```python
from build123d import *

# Parameters (mm, degrees)
SKETCH1_W                = 50
SKETCH1_H                = 35.6
BOSS_EXTRUDE2_DEPTH      = 15
SKETCH9_W                = 2.17
SKETCH9_H                = 25.6
CUT_EXTRUDE1_DEPTH       = 10.3
SKETCH7_R                = 1.32
CUT_EXTRUDE2_DEPTH       = 34.770899441
SKETCH10_R               = 0.81
CUT_EXTRUDE3_DEPTH       = 8
BOSS_EXTRUDE3_DEPTH      = 0.3
BOSS_EXTRUDE3_DEPTH_BACK = 1.87


with BuildPart() as part:
    # Sketch1 → Boss-Extrude2 (new body)
    with BuildSketch(Plane(origin=(0, 0, 0), x_dir=(1, 0, 0), z_dir=(0, 1, 0))):
        Rectangle(SKETCH1_W, SKETCH1_H)
    extrude(amount=-BOSS_EXTRUDE2_DEPTH)

    # Sketch9 → Cut-Extrude1 (cut)
    with BuildSketch(Plane(origin=(0, 0, 0), x_dir=(1, 0, 0), z_dir=(0, 1, 0))):
        with Locations((-0.785, 0)):
            Rectangle(SKETCH9_W, SKETCH9_H)
    extrude(amount=-CUT_EXTRUDE1_DEPTH, mode=Mode.SUBTRACT)

    # Sketch7 → Cut-Extrude2 (cut, through all)
    with BuildSketch(Plane(origin=(-1.180715955, -3.243990424, 0), x_dir=(-0.9396926207859082, 0.3420201433256691, 0), z_dir=(-0.3420201433256691, -0.9396926207859082, 0))):
        with Locations(Location((-3.68818129, 10.1, 0), (0, 0, 180))):
            Circle(SKETCH7_R)
        with Locations(Location((-3.68818129, 6.46, 0), (0, 0, 180))):
            Circle(SKETCH7_R)
        with Locations(Location((-3.68818129, 2.82, 0), (0, 0, 180))):
            Circle(SKETCH7_R)
        with Locations(Location((-3.68818129, -0.82, 0), (0, 0, 180))):
            Circle(SKETCH7_R)
        with Locations(Location((-3.68818129, -6.46, 0), (0, 0, 180))):
            Circle(SKETCH7_R)
        with Locations(Location((-3.68818129, -10.1, 0), (0, 0, 180))):
            Circle(SKETCH7_R)
    extrude(amount=-CUT_EXTRUDE2_DEPTH, mode=Mode.SUBTRACT)

    # Sketch10 → Cut-Extrude3 (cut)
    with BuildSketch(Plane(origin=(-1.180715955, -3.243990424, 0), x_dir=(-0.9396926207859082, 0.3420201433256691, 0), z_dir=(-0.3420201433256691, -0.9396926207859082, 0))):
        with Locations(Location((-3.68818129, -10.1, 0), (0, 0, 180))):
            Circle(SKETCH10_R)
        with Locations(Location((-3.68818129, -6.46, 0), (0, 0, 180))):
            Circle(SKETCH10_R)
        with Locations(Location((-3.68818129, -0.82, 0), (0, 0, 180))):
            Circle(SKETCH10_R)
        with Locations(Location((-3.68818129, 2.82, 0), (0, 0, 180))):
            Circle(SKETCH10_R)
        with Locations(Location((-3.68818129, 6.46, 0), (0, 0, 180))):
            Circle(SKETCH10_R)
        with Locations(Location((-3.68818129, 10.1, 0), (0, 0, 180))):
            Circle(SKETCH10_R)
    extrude(amount=CUT_EXTRUDE3_DEPTH, mode=Mode.SUBTRACT)

    # Sketch11 → Boss-Extrude3 (add, two sides: drawn at the far end of the back side and taken through both)
    with BuildSketch(Plane(origin=(0, 0, 0), x_dir=(0, 0, -1), z_dir=(1, 0, 0)).offset(-BOSS_EXTRUDE3_DEPTH_BACK)):
        Polygon((-4.40036814, -10.3), (-2.87963186, -10.3), (-3.367024207, -1), (-3.912975793, -1), align=None)
    extrude(amount=BOSS_EXTRUDE3_DEPTH + BOSS_EXTRUDE3_DEPTH_BACK)


solid = part.part
```
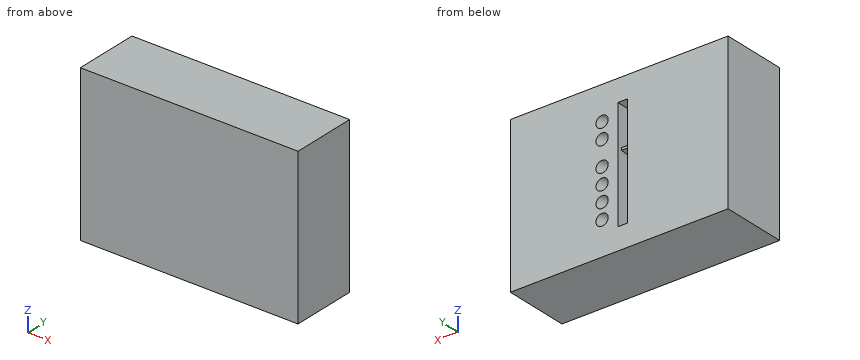
CAD build for the part. Positions are in the model's coordinates, mm. Coordinates: 2 decimals unless noted, no trailing zeros.
(1) Cut at A-A, the plane y = -7. Count the separate pieces of the cut face and the enclosed holes in it, and give its area (3 significant figures).
(2) Drill centre lines: probe 1 along X at (y, z) = (-2, -8); probe 2 along X at (y, z) = (-0.25, 7); probe 3 along X at (y, z) = (-1.75, -10). Where is each one in solid material? Low to high.
(3) Flat gauge pins, fed straight in: pin 1 (0.7 mm diameter, centred on x = -1, z = -1.5, fed in from +Y); pin 2 (2.5 mm diameter, centred on x = -0.5, z = 7.5, fed in from +Y); pin 3 (0.6 mm diameter, centred on x = -1, z = 3.5, fed in from +Y). Where does each tip first touch, or does it go through?
Geometry says:
1. separate pieces: 1
1. enclosed holes: 8
1. area: 1,710 mm2
2. probe 1: x = -25 to -1.87, 0.3 to 25
2. probe 2: x = -25 to -1.87, 0.3 to 2.55, 5.12 to 25
2. probe 3: x = -25 to -1.87, 0.3 to 1.89, 4.69 to 25
3. pin 1: stops at y = -10.3
3. pin 2: stops at y = 0
3. pin 3: stops at y = -1
